Geometry check sheet. Reference: drawing and pictorial views, mm from the part's lowest x, y, z. Give positions to 0.01 mm unless a question says otherwise; leave off trailing zeros. Loops run counter-clockwise (first coordinate to the right, second up) from the corner with the lowest first, then second, coordinate; pieces in that order, holes last. Notation, with made-up numbers: M 55.5,51 L 107.5,51 A23 cw 107.5,63 Z; hole C 21.5,31 d11. An arc over 180 degrees is marked long. Use CSV: the item, a comma, the result in double quotes.
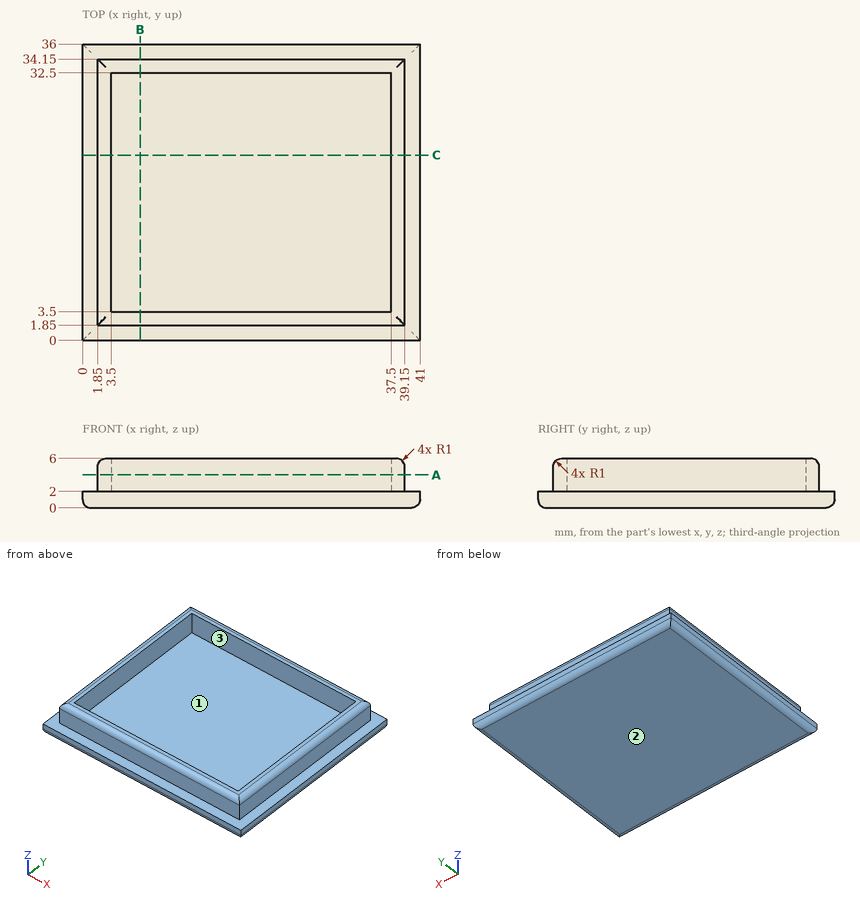
(1) Section check A-A on z = 4. Record the cut outline in (x, y).
Calculated:
outline,"M 1.85,1.85 L 39.15,1.85 L 39.15,34.15 L 1.85,34.15 Z; hole M 3.5,3.5 L 37.5,3.5 L 37.5,32.5 L 3.5,32.5 Z"
(2) Depth check by flat-ended pin: pin 1 Ø0.9 at (x, z) = (24.5, 3.5) entering from -Y; pin 2 Ø2 at (y, z) = (12.5, 4) entering from -X; pin 3 Ø1.5 at (x, z) = (23.5, 4) entering from +Y. Enter the tip coordinate at first touch or a pass-through.
Calculated:
pin 1,"stops at y = 1.85"
pin 2,"stops at x = 1.85"
pin 3,"stops at y = 34.15"
(3) Mould release check, pull along Y, two halves, no side actions. Record for the marked faces 1, 2 and 3: released by +Y, released by -Y, zero draft, split by the parting line, or undercut.
Calculated:
face 1,"undercut"
face 2,"zero draft"
face 3,"undercut"
(4) Section check B-B on x = 7. Record the cut outline in (y, z), plus the area to 3 significant figures.
Calculated:
outline,"M 0,1 A1 ccw 1,0 L 35,0 A1 ccw 36,1 L 36,2 L 34.15,2 L 34.15,5 A1 ccw 33.15,6 L 32.5,6 L 32.5,2 L 3.5,2 L 3.5,6 L 2.85,6 A1 ccw 1.85,5 L 1.85,2 L 0,2 Z"
area,"84.3 mm²"
(5) Scan lines: L1, parallel to Y at x = 33.5, z = 2.75; L2, parallel to X at y = 25, z = 2.5; L3, parallel to Z at x = 23.5, y = 29. Record each from-to range of solid material in increasing order. Write a range as from..to.
Calculated:
L1,"y = 1.85..3.5, 32.5..34.15"
L2,"x = 1.85..3.5, 37.5..39.15"
L3,"z = 0..2"
(6) Section check C-C on y = 22.5. Record the cut outline in (x, z), plus the area to 3 significant figures.
Calculated:
outline,"M 0,1 A1 ccw 1,0 L 40,0 A1 ccw 41,1 L 41,2 L 39.15,2 L 39.15,5 A1 ccw 38.15,6 L 37.5,6 L 37.5,2 L 3.5,2 L 3.5,6 L 2.85,6 A1 ccw 1.85,5 L 1.85,2 L 0,2 Z"
area,"94.3 mm²"
